The listing builds one solid part. Answer for the finished solid, in the listing's coordinates (mm). Coordinates: 2 decimals unless noted, no trailing zeros. Write each loop counter-clockwise with the first axis right and the second up, starting at its lowest first coordinate (ties: lowest second). Pieces come first, ordered by that corner, then holes.
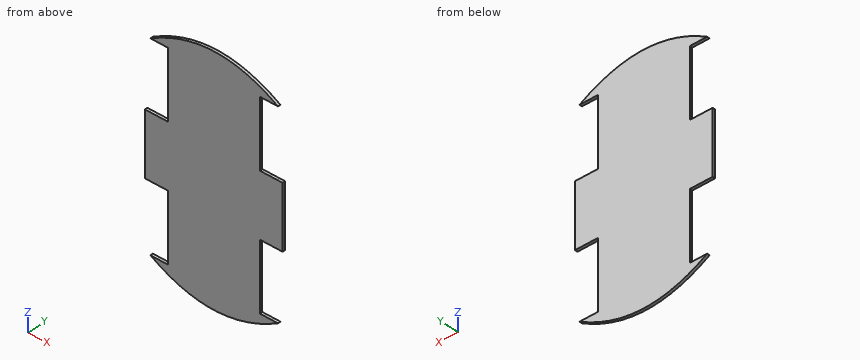
from build123d import *

# Parameters (mm, degrees)
EXTRUDE_1_DEPTH = 3


with BuildPart() as part:
    # 草图1 → 凸台-拉伸1 (new body)
    with BuildSketch(Plane(origin=(0, 0, 0), x_dir=(1, 0, 0), z_dir=(0, 1, 0))):
        with BuildLine():
            Line((-49.987744463, 0), (-49.987744463, 75))
            Line((-49.987744463, 75), (-69.064059337, 75))
            add(Edge.make_bspline(
                [(-69.064059337, 75), (0.777424166, 117.582810978), (70.935940663, 75)],
                knots=[0, 0, 0, 1, 1, 1], degree=2))
            Line((70.935940663, 75), (50.935940663, 75))
            Line((50.935940663, 75), (50.935940663, 0))
            Line((50.935940663, 0), (75.935940663, 0))
            Line((75.935940663, 0), (75.935940663, -70))
            Line((75.935940663, -70), (50.935940663, -70))
            Line((50.935940663, -70), (50.935940663, -145))
            Line((50.935940663, -145), (70.935940663, -145))
            add(Edge.make_bspline(
                [(-69.064059337, -145), (0.777424166, -187.582810978), (70.935940663, -145)],
                knots=[0, 0, 0, 1, 1, 1], degree=2))
            Line((-69.064059337, -145), (-49.987744463, -145))
            Line((-49.987744463, -145), (-49.987744463, -70))
            Line((-49.987744463, -70), (-74.987744463, -70))
            Line((-74.987744463, -70), (-74.987744463, 0))
            Line((-74.987744463, 0), (-49.987744463, 0))
        make_face()
    extrude(amount=EXTRUDE_1_DEPTH)


solid = part.part
Q1. Find the intervals of material crossed by probe 1 along Z at (x, y) = (-68.5, 2.45); probe 2 along Z at (x, y) = (-55, 1.9); probe 3 along X at (y, z) = (0.3, -50), in increasing order.
Answers below:
probe 1: z = -75.34 to -75, 0 to 70, 145 to 145.34
probe 2: z = -82.71 to -75, 0 to 70, 145 to 152.71
probe 3: x = -49.99 to 50.94
Q2. The part is cut by section A-A, the plane x = -52.5. State how many separate pieces and enclosed holes the cut face has, then the cut area to 3 significant figures.
Answers below:
separate pieces: 3
enclosed holes: 0
area: 263 mm2
Q3. The part is cut by section B-B, the plane z = -32. Write down the section's boundary in (x, y), then the cut area to 3 significant figures.
Answers below:
outline: (-49.99, 0) - (50.94, 0) - (50.94, 3) - (-49.99, 3) - close
area: 303 mm2
Q4. Given pin 1 (0.9 mm diameter, centred on y = 1, z = 116, fed in from -X); pin 2 (0.9 mm diameter, centred on x = 66, y = 1, fed in from +Z); pin 3 (1.5 mm diameter, centred on x = -62.5, y = 1, fed in from -Z), each flat-ended and moving along its own axis, determine where each tip first touches the part or whether it passes through.
Answers below:
pin 1: stops at x = -49.99
pin 2: stops at z = 148.14
pin 3: stops at z = -79.23
